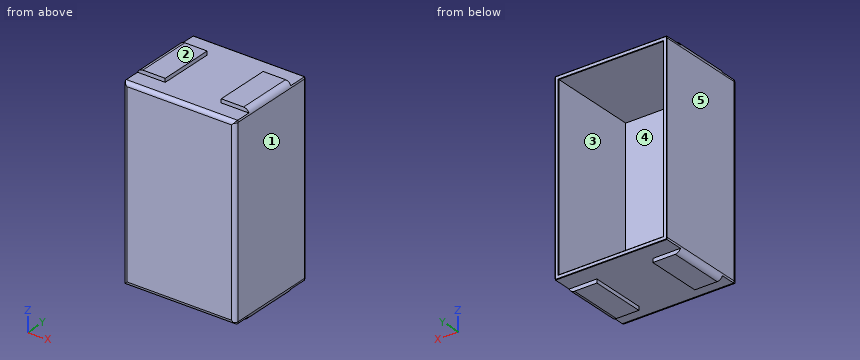
from build123d import *

# Parameters (mm, degrees)
SKETCH2_W            = 60
SKETCH2_H            = 100
BOSS_EXTRUDE1_DEPTH  = 50
SKETCH3_W            = 56
SKETCH3_H            = 96
CUT_EXTRUDE1_DEPTH   = 48
SKETCH4_W            = 15
SKETCH4_H            = 30
BOSS_EXTRUDE2_DEPTH  = 2
FILLET1_R            = 3
FILLET1_OF_MIRROR1_R = 3
FILLET2_R            = 2
FILLET3_R            = 0.25


with BuildPart() as part:
    # Sketch2 → Boss-Extrude1 (new body)
    with BuildSketch(Plane(origin=(0, 0, 0), x_dir=(1, 0, 0), z_dir=(0, 1, 0))):
        Rectangle(SKETCH2_W, SKETCH2_H)
    extrude(amount=BOSS_EXTRUDE1_DEPTH)

    # Sketch3 → Cut-Extrude1 (cut)
    with BuildSketch(Plane(origin=(0, 50, 0), x_dir=(1, 0, 0), z_dir=(0, 1, 0))):
        Rectangle(SKETCH3_W, SKETCH3_H)
    extrude(amount=-CUT_EXTRUDE1_DEPTH, mode=Mode.SUBTRACT)

    # Sketch4 → Boss-Extrude2 (add)
    with BuildSketch(Plane(origin=(0, 0, -50), x_dir=(-1, 0, 0), z_dir=(0, 0, -1))):
        with Locations((-22.5, 25)):
            Rectangle(SKETCH4_W, SKETCH4_H)
        with Locations((22.5, 25)):
            Rectangle(SKETCH4_W, SKETCH4_H)
    boss_extrude2 = extrude(amount=BOSS_EXTRUDE2_DEPTH)

    # Fillet1
    fillet1_edges = [part.edges().sort_by_distance(p)[0] for p in [
        (30, 25, -52),
        (-30, 25, -52),
    ]]
    fillet(fillet1_edges, radius=FILLET1_R)

    # Mirror1: Boss-Extrude2 across plane
    add(boss_extrude2.mirror(Plane.XY))

    # Fillet1 of Mirror1
    fillet1_of_mirror1_edges = [part.edges().sort_by_distance(p)[0] for p in [
        (30, 25, 52),
        (-30, 25, 52),
    ]]
    fillet(fillet1_of_mirror1_edges, radius=FILLET1_OF_MIRROR1_R)

    # Fillet2
    # the kernel refuses this fillet: 2 mm, written as the material it takes off along each edge
    with BuildSketch(Plane(origin=(34.828427125, 0, -50), x_dir=(0, 0, 1), z_dir=(-1, 0, 0)), Plane(origin=(-34.828427125, 0, 50), x_dir=(0, 0, -1), z_dir=(1, 0, 0))) as fillet2_piece_1:
        with BuildLine():
            CenterArc((FILLET2_R, FILLET2_R), FILLET2_R, 180, 90)
            Line((0, FILLET2_R), (0, 0))
            Line((0, 0), (FILLET2_R, 0))
        make_face()
    extrude(amount=69.656854249, mode=Mode.SUBTRACT)
    with BuildSketch(Plane(origin=(-30, 0, -49), x_dir=(0, 1, 0), z_dir=(0, 0, 1))) as fillet2_piece_2:
        with BuildLine():
            CenterArc((FILLET2_R, -FILLET2_R), FILLET2_R, 90, 90)
            Line((0, -FILLET2_R), (0, 0))
            Line((0, 0), (FILLET2_R, 0))
        make_face()
    extrude(amount=98, mode=Mode.SUBTRACT)
    with BuildSketch(Plane(origin=(30, 0, 49), x_dir=(-1, 0, 0), z_dir=(0, 0, -1))) as fillet2_piece_3:
        with BuildLine():
            CenterArc((FILLET2_R, FILLET2_R), FILLET2_R, 180, 90)
            Line((0, FILLET2_R), (0, 0))
            Line((0, 0), (FILLET2_R, 0))
        make_face()
    extrude(amount=98, mode=Mode.SUBTRACT)
    with BuildSketch(Plane(origin=(27, 0, 49), x_dir=(1, 0, 0), z_dir=(0, 0, -1))) as fillet2_piece_4:
        with BuildLine():
            CenterArc((3 - FILLET2_R, -FILLET2_R), FILLET2_R, 0, 90)
            Line((3, -FILLET2_R), (3, 0))
            Line((3, 0), (3 - FILLET2_R, 0))
        make_face()
    revolve(axis=Axis((27, 0, 49), (0, -1, 0)), revolution_arc=114.9659815, mode=Mode.SUBTRACT)
    with BuildSketch(Plane(origin=(27, 0, -49), x_dir=(1, 0, 0), z_dir=(0, 0, 1))) as fillet2_piece_5:
        with BuildLine():
            CenterArc((3 - FILLET2_R, FILLET2_R), FILLET2_R, 270, 90)
            Line((3, FILLET2_R), (3, 0))
            Line((3, 0), (3 - FILLET2_R, 0))
        make_face()
    revolve(axis=Axis((27, 0, -49), (0, 1, 0)), revolution_arc=114.9659815, mode=Mode.SUBTRACT)
    with BuildSketch(Plane(origin=(-27, 0, -49), x_dir=(-1, 0, 0), z_dir=(0, 0, 1))) as fillet2_piece_6:
        with BuildLine():
            CenterArc((3 - FILLET2_R, -FILLET2_R), FILLET2_R, 0, 90)
            Line((3 - FILLET2_R, 0), (3, 0))
            Line((3, 0), (3, -FILLET2_R))
        make_face()
    revolve(axis=Axis((-27, 0, -49), (0, -1, 0)), revolution_arc=114.9659815, mode=Mode.SUBTRACT)
    with BuildSketch(Plane(origin=(-27, 0, 49), x_dir=(-1, 0, 0), z_dir=(0, 0, -1))) as fillet2_piece_7:
        with BuildLine():
            CenterArc((3 - FILLET2_R, FILLET2_R), FILLET2_R, 270, 90)
            Line((3 - FILLET2_R, 0), (3, 0))
            Line((3, 0), (3, FILLET2_R))
        make_face()
    revolve(axis=Axis((-27, 0, 49), (0, 1, 0)), revolution_arc=114.9659815, mode=Mode.SUBTRACT)

    # Fillet3
    fillet3_edges = [part.edges().sort_by_distance(p)[0] for p in [
        (0, 50, 50),
        (-29.956795679, 50, 49.507305936),
        (29.956795679, 50, 49.507305936),
        (28, 50, 0),
        (0, 50, -48),
        (-28, 50, 0),
        (0, 50, 48),
        (0, 50, -50),
        (-30, 50, 0),
        (-29.956795679, 50, -49.507305936),
        (29.956795679, 50, -49.507305936),
        (30, 50, 0),
    ]]
    fillet(fillet3_edges, radius=FILLET3_R)


solid = part.part
Verification items for the finished model (mm, model axes). Face numbers are marked on the shaded views. A direction names the side the tool comes from. Round coordinates to 2 decimals unless told otherwise and drop trailing zeros. Write each loop counter-clockwise with the first axis right and the second up, starting at its lowest first coordinate (ties: lowest second). Pieces come first, ordered by that corner, then holes.
(1) Section check D-D (y = 21). Enter the section's corners in (x, z), plus the area to 3 significant figures.
Returned:
outline: (-30, -49) arc R3 ccw to (-27, -52) - (-15, -52) - (-15, -50) - (15, -50) - (15, -52) - (27, -52) arc R3 ccw to (30, -49) - (30, 49) arc R3 ccw to (27, 52) - (15, 52) - (15, 50) - (-15, 50) - (-15, 52) - (-27, 52) arc R3 ccw to (-30, 49) - close; hole (-28, -48) - (28, -48) - (28, 48) - (-28, 48) - close
area: 736 mm2
(2) Mould release check, pull along Z, two halves, no side actions. Record for the marked faces 1, 2 and 3: pulls with the +Z half, pulls with the -Z half, needs draft (parallel to the pull), parting line crosses it, or undercut.
Returned:
face 1: needs draft
face 2: pulls with the +Z half
face 3: undercut
(3) Access from +Z, -Z, +X, -X, +Y, -Y to the whole of each face (thin tool, end or side, straight path). Record for the marked faces 4 and 5.
Returned:
face 4: +Y
face 5: +Z, -Z, -X, +Y, -Y
(4) Depth check by flat-ended pin: pin 1 Ø4 at (x, z) = (-8.5, 12) entering from +Y; pin 2 Ø0.6 at (y, z) = (19, -51) entering from +X; pin 3 Ø2 at (x, z) = (22, -50.5) entering from -Y. Enter the tip coordinate at first touch or a pass-through.
Returned:
pin 1: stops at y = 2
pin 2: stops at x = 29.47
pin 3: stops at y = 0.68
(5) Section check A-A (y = 4.5). Enter the section's corners in (x, z), plus the area to 3 significant figures.
Returned:
outline: (-30, -49) arc R3 ccw to (-29.83, -50) - (29.83, -50) arc R3 ccw to (30, -49) - (30, 49) arc R3 ccw to (29.83, 50) - (-29.83, 50) arc R3 ccw to (-30, 49) - close; hole (-28, -48) - (28, -48) - (28, 48) - (-28, 48) - close
area: 624 mm2
(6) Material ranges on line 1 (X direction, y = 8, z = 34); line 2 (Z direction, x = -6.5, y = 48); line 3 (Z direction, x = -16, y = 27.5), recorded low to high.
Returned:
line 1: x = -30 to -28, 28 to 30
line 2: z = -50 to -48, 48 to 50
line 3: z = -52 to -48, 48 to 52
(7) Section check B-B (z = 33.5). Enter the section's corners in (x, y).
Returned:
outline: (-30, 2) arc R2 ccw to (-28, 0) - (28, 0) arc R2 ccw to (30, 2) - (30, 49.75) arc R0.25 ccw to (29.75, 50) - (28.25, 50) arc R0.25 ccw to (28, 49.75) - (28, 2) - (-28, 2) - (-28, 49.75) arc R0.25 ccw to (-28.25, 50) - (-29.75, 50) arc R0.25 ccw to (-30, 49.75) - close
(8) Section check C-C (x = 23.5). Enter the section's corners in (y, z).
Returned:
outline: (0, -48) arc R2 ccw to (2, -50) - (10, -50) - (10, -52) - (40, -52) - (40, -50) - (49.75, -50) arc R0.25 ccw to (50, -49.75) - (50, -48.25) arc R0.25 ccw to (49.75, -48) - (2, -48) - (2, 48) - (49.75, 48) arc R0.25 ccw to (50, 48.25) - (50, 49.75) arc R0.25 ccw to (49.75, 50) - (40, 50) - (40, 52) - (10, 52) - (10, 50) - (2, 50) arc R2 ccw to (0, 48) - close
